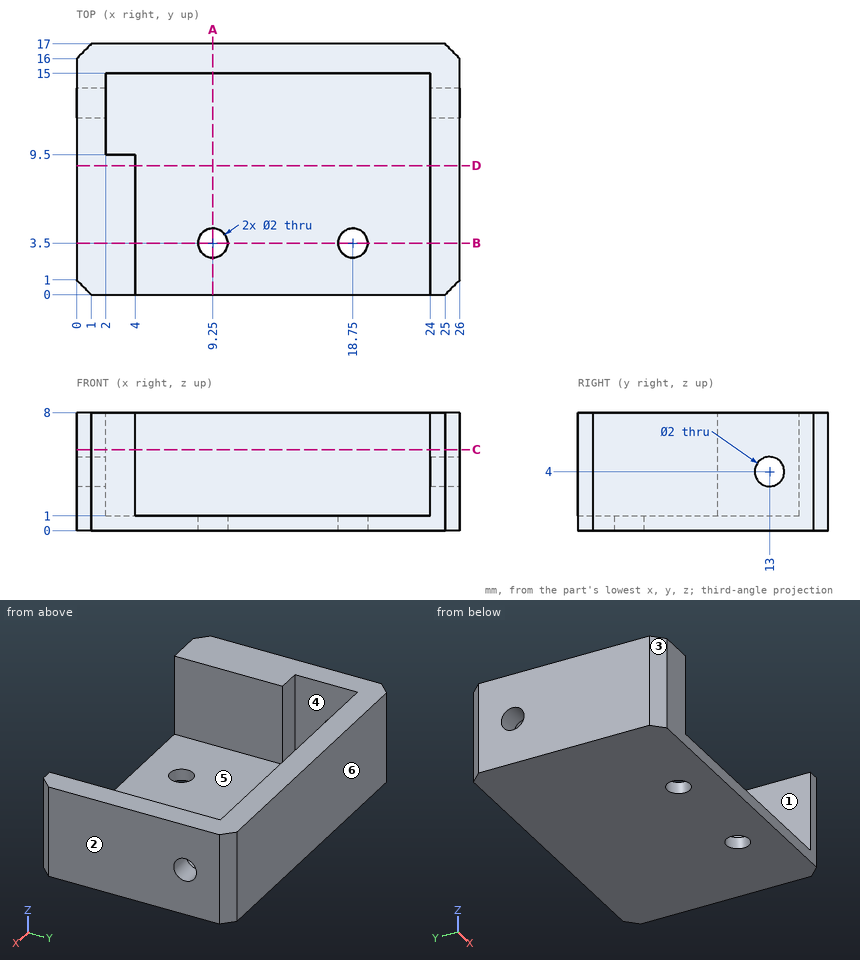
Study the drawing (mm; zero at the part's minimum x, y, z) and answer. A direction names the side the tool comes from. Give positions to 0.01 mm unless a question says otherwise; leave off trailing zeros. Write each loop counter-clockwise with the first axis right and the second up, starting at its lowest first coordinate (ties: lowest second). Pieces come first, ordered by that corner, then holes.
(1) The part is cut by section C-C on z = 5.5. Write down the section's boundary in (x, y).
Final values:
outline: (0, 1) - (1, 0) - (4, 0) - (4, 9.5) - (2, 9.5) - (2, 15) - (24, 15) - (24, 0) - (25, 0) - (26, 1) - (26, 16) - (25, 17) - (1, 17) - (0, 16) - close
(2) The part is cut by section A-A on x = 9.25. Write down the section's boundary in (y, z).
Final values:
outline: (0, 0) - (2.5, 0) - (2.5, 1) - (0, 1) - close; (4.5, 0) - (17, 0) - (17, 8) - (15, 8) - (15, 1) - (4.5, 1) - close
(3) The part is cut by section D-D on y = 8.75. Write down the section's boundary in (x, z).
Final values:
outline: (0, 0) - (26, 0) - (26, 8) - (24, 8) - (24, 1) - (4, 1) - (4, 8) - (0, 8) - close
(4) Straight lines are drawn through the part: line 1 (X direction, y = 3.5, z = 0.2); line 2 (X direction, y = 2.5, z = 7.75); line 3 (X direction, y = 11, z = 5.5). For each, find the intervals that lie inside material, in ascending order.
Final values:
line 1: x = 0 to 8.25, 10.25 to 17.75, 19.75 to 26
line 2: x = 0 to 4, 24 to 26
line 3: x = 0 to 2, 24 to 26
(5) The mould has two halves that part along X. Classify the marked faces 3, 4, 5 and 6: pulls with the +X half, pulls with the -X half, needs draft (parallel to the pull), parting line crosses it, or undercut.
Final values:
face 3: pulls with the -X half
face 4: undercut
face 5: undercut
face 6: needs draft
(6) Which of the six approach directions +Z, -Z, +X, -X, +Y, -Y give full straight-line access (tool end or side, diameter ignored) to the marked faces 1 and 2?
Final values:
face 1: +Z, -Y
face 2: +Z, -Z, +X, +Y, -Y
(7) Flat-ended cylindrical pins translate along their axes: pin 1 Ø2 at (y, z) = (9, 5) entering from -X; pin 2 Ø1.2 at (y, z) = (13, 4) entering from +X; pin 3 Ø2 at (x, z) = (11.5, 5.5) entering from -Y; pin 4 Ø7.5 at (x, y) = (8, 10.5) entering from +Z. Find the tip coordinate at first contact, or state that the pin passes through.
Final values:
pin 1: stops at x = 0
pin 2: passes through
pin 3: stops at y = 15
pin 4: stops at z = 1
(8) The part is cut by section B-B on y = 3.5. Write down the section's boundary in (x, z), plus the area to 3 significant figures.
Final values:
outline: (0, 0) - (8.25, 0) - (8.25, 1) - (4, 1) - (4, 8) - (0, 8) - close; (10.25, 0) - (17.75, 0) - (17.75, 1) - (10.25, 1) - close; (19.75, 0) - (26, 0) - (26, 8) - (24, 8) - (24, 1) - (19.75, 1) - close
area: 64.0 mm2
